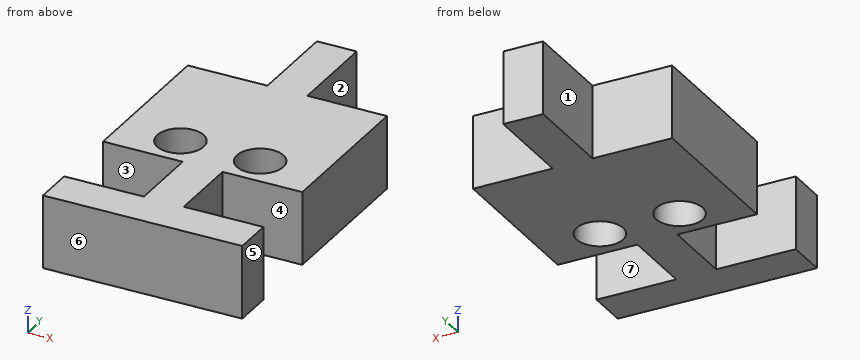
from build123d import *

# Parameters (mm, degrees)
EXTRUDE_1_DEPTH     = 5.5
SKETCH_2_R          = 1.75
CUT_EXTRUDE_1_DEPTH = 30.030156734


with BuildPart() as part:
    # ｽｹｯﾁ1 → ﾎﾞｽ - 押し出し1 (new body)
    with BuildSketch(Plane.XY):
        Polygon((1.5, -7), (7.5, -7), (7.5, -19), (1.5, -19), (1.5, -24.5), (7.5, -24.5), (7.5, -27.5), (-7.5, -27.5), (-7.5, -24.5), (-1.5, -24.5), (-1.5, -19), (-7.5, -19), (-7.5, -7), (-1.5, -7), (-1.5, 0), (1.5, 0), align=None)
    extrude(amount=EXTRUDE_1_DEPTH)

    # ｽｹｯﾁ2 → ｶｯﾄ - 押し出し1 (cut, through all)
    with BuildSketch(Plane.XY.offset(5.5)):
        with Locations((-3, -16.5)):
            Circle(SKETCH_2_R)
        with Locations((3, -16.5)):
            Circle(SKETCH_2_R)
    extrude(amount=-CUT_EXTRUDE_1_DEPTH, mode=Mode.SUBTRACT)


solid = part.part
Here's how the part is built. I have some questions about the finished solid (model axes, mm). Face numbers are marked on the shaded views. A direction names the side the tool comes from. Coordinates: 2 decimals unless noted, no trailing zeros. Order: outer loops, then holes, each group sorted by start corner. A loop starts at its lowest first (then second) coordinate and runs counter-clockwise, first axis right, second up. Notation, with made-up numbers: (26.25, -25) -> (32.25, -25) arc R30 ccw to (32.25, 0) -> close; hole circle Ø2 at (58.5, 72). An arc over 180 degrees is marked (long way). Answer in a Markdown table with one row per item.
(1) Please list where these lines run through material, in increasing order: probe 1 along Y at (x, z) = (-3, 3.4); probe 2 along Y at (x, z) = (-5.75, 4.05); probe 3 along Y at (x, z) = (-4.25, 4.05).
Answer key:
| item | result |
|---|---|
| probe 1 | -27.5 to -24.5, -19 to -18.25, -14.75 to -7 |
| probe 2 | -27.5 to -24.5, -19 to -7 |
| probe 3 | -27.5 to -24.5, -19 to -17.72, -15.28 to -7 |
(2) I want a section at C-C on x = -3. List the corners of the cut face in (y, z) for me, then the cut area to 4 significant figures.
Answer key:
| item | result |
|---|---|
| outline | (-27.5, 0) -> (-24.5, 0) -> (-24.5, 5.5) -> (-27.5, 5.5) -> close; (-19, 0) -> (-18.25, 0) -> (-18.25, 5.5) -> (-19, 5.5) -> close; (-14.75, 0) -> (-7, 0) -> (-7, 5.5) -> (-14.75, 5.5) -> close |
| area | 63.25 mm^2 |
(3) I want a section at B-B on z = 1.1. List the corners of the cut face in (x, y) for me, then the cut area to 3 significant figures.
Answer key:
| item | result |
|---|---|
| outline | (-7.5, -27.5) -> (7.5, -27.5) -> (7.5, -24.5) -> (1.5, -24.5) -> (1.5, -19) -> (7.5, -19) -> (7.5, -7) -> (1.5, -7) -> (1.5, 0) -> (-1.5, 0) -> (-1.5, -7) -> (-7.5, -7) -> (-7.5, -19) -> (-1.5, -19) -> (-1.5, -24.5) -> (-7.5, -24.5) -> close; hole circle Ø3.5 at (-3, -16.5); hole circle Ø3.5 at (3, -16.5) |
| area | 243 mm^2 |
(4) Thinking about a two-plate mould opening in Y: for the marked faces 5, 6 and 7, which applies, +Y half, -Y half, draft (parallel to the pull), parting line (faces both ways), or undercut?
Answer key:
| item | result |
|---|---|
| face 5 | draft |
| face 6 | -Y half |
| face 7 | undercut |
(5) I want a section at A-A on x = 6. List the corners of the cut face in (y, z) for me, then the cut area to 3 significant figures.
Answer key:
| item | result |
|---|---|
| outline | (-27.5, 0) -> (-24.5, 0) -> (-24.5, 5.5) -> (-27.5, 5.5) -> close; (-19, 0) -> (-7, 0) -> (-7, 5.5) -> (-19, 5.5) -> close |
| area | 82.5 mm^2 |
(6) I want a section at D-D on y = -4.25. List the corners of the cut face in (x, z) for me, then the cut area to 3 significant figures.
Answer key:
| item | result |
|---|---|
| outline | (-1.5, 0) -> (1.5, 0) -> (1.5, 5.5) -> (-1.5, 5.5) -> close |
| area | 16.5 mm^2 |
(7) Will these pins go through, and if not, where does the flat tip stop? pin 1 Ø3 at (y, z) = (-22.5, 1.5) entering from -X; pin 2 Ø1.6 at (y, z) = (-2.5, 3.5) entering from +X; pin 3 Ø1.6 at (x, z) = (4.5, 3.5) entering from +Y.
Answer key:
| item | result |
|---|---|
| pin 1 | x = -1.5 |
| pin 2 | x = 1.5 |
| pin 3 | y = -7 |
(8) On a 3-axis mill with a long thin cutter (end or side, diameter ignored), from which of +Z, -Z, +X, -X, +Y, -Y can I reach the whole of each face in a straight line? I mean the marked faces 1, 2, 3 and 4. Say none if no direction works.
Answer key:
| item | result |
|---|---|
| face 1 | +Z, -Z, -X, +Y |
| face 2 | +Z, -Z, +X, +Y |
| face 3 | +Z, -Z, -X |
| face 4 | +Z, -Z, +X |
